The listing builds one solid part. Answer for the finished solid, in the listing's coordinates (mm). A direction names the side the tool comes from. Give positions to 0.01 mm unless a question says otherwise; leave off trailing zeros. Order: outer loops, then holes, each group sorted by start corner. A loop starts at its lowest first (then second) coordinate and runs counter-clockwise, first axis right, second up. Notation, with made-up numbers: (79.25, 16.25) - (130.25, 16.25) arc R29 ccw to (130.25, 46.25) - close; hole circle Ø7 at (13.25, 4). An arc over 180 degrees is marked (long way). Answer as a JSON object with one key per item and string values. Group by question number.
Q1. A cutting plane is placed at B-B, the plane y = 245.5. Give the vertices of the cut face in (x, z) (3 decimals), and give its area (3 significant figures).
Q2. Given pin 1 (6 mm diameter, centred on y = -110.93, z = 0, fed in from -X), flat-ended and moving along its own axis, determine where the tip first touches the part or whether it passes through.
Q3. For faces 1 (the face through (0, 5, 12.7)), 2 (the face through (22.225, 5, 0)), determine the directions among +Z, -Z, +X, -X, +Y, -Y from which every point of the face is accessible in a straight line to the end or side of a thin tool.
Q4. The mould has two halves that part along X. Classify faces 3 (the face through (0, -381, -10)), 4 (the face through (25.4, 5, 0)), 5 (the face through (-22.225, 5, 0)): released by +X, released by -X, zero draft, split by the parting line, or undercut.
Q5. A cutting plane is placed at A-A, the plane x = 1. Give the vertices of the cut face in (y, z) (3 decimals).
Q6. Consider line 1 (Y direction, x = -12.7, z = -10.75); line 2 (Z direction, x = 20, y = 268) (3 decimals); line 3 (X direction, y = 231.5, z = 1.5) (3 decimals). Determine where each line is inside the solid, lowest interval first.
from build123d import *

# Parameters (mm, degrees)
SKETCH1_W               = 50.8
SKETCH1_H               = 25.4
BOSS_EXTRUDE1_DEPTH     = 381
SHELL1_T                = -3.175
SKETCH4_R               = 2.38125
CUT_EXTRUDE1_DEPTH      = 385.581499815
CUT_EXTRUDE2_DEPTH      = 383.689587002
CUT_EXTRUDE2_DEPTH_BACK = 383.689587002
SKETCH5_R               = 2.38125


with BuildPart() as part:
    # Sketch1 → Boss-Extrude1 (new, symmetric)
    with BuildSketch(Plane(origin=(0, 0, 0), x_dir=(1, 0, 0), z_dir=(0, 1, 0))):
        Rectangle(SKETCH1_W, SKETCH1_H)
    extrude(amount=BOSS_EXTRUDE1_DEPTH, both=True)

    # Shell1
    shell1_openings = [part.faces().sort_by_distance(p)[0] for p in [
        (0, 381, 0),
        (0, -381, 0),
    ]]
    offset(amount=SHELL1_T, openings=shell1_openings, kind=Kind.INTERSECTION)

    # Sketch4 → Cut-Extrude1 (cut, through all)
    with BuildSketch(Plane(origin=(25.4, 0, 0), x_dir=(0, 0, -1), z_dir=(1, 0, 0))):
        with Locations((0, 110.9345)):
            Circle(SKETCH4_R)
        with Locations((0, 98.2345)):
            Circle(SKETCH4_R)
        with Locations((0, 85.5345)):
            Circle(SKETCH4_R)
        with Locations(Location((0, -85.5345, 0), (0, 0, 180))):
            Circle(SKETCH4_R)
        with Locations(Location((0, -98.2345, 0), (0, 0, 180))):
            Circle(SKETCH4_R)
        with Locations(Location((0, -110.9345, 0), (0, 0, 180))):
            Circle(SKETCH4_R)
        with Locations((0, -12.7)):
            Circle(SKETCH4_R)
        with Locations((0, -38.1)):
            Circle(SKETCH4_R)
        with Locations(Location((0, 38.1, 0), (0, 0, 180))):
            Circle(SKETCH4_R)
        with Locations(Location((0, 12.7, 0), (0, 0, 180))):
            Circle(SKETCH4_R)
    extrude(amount=-CUT_EXTRUDE1_DEPTH, mode=Mode.SUBTRACT)

    # Sketch5 → Cut-Extrude2 (cut, two sides: drawn at the far end of the back side and taken through both)
    with BuildSketch(Plane.XY.offset(12.7).offset(-CUT_EXTRUDE2_DEPTH_BACK)):
        with Locations((-12.7, 368.3)):
            Circle(SKETCH5_R)
        with Locations((12.7, 368.3)):
            Circle(SKETCH5_R)
        with Locations((12.7, 342.9)):
            Circle(SKETCH5_R)
        with Locations((-12.7, 342.9)):
            Circle(SKETCH5_R)
        with Locations((-12.7, -342.9)):
            Circle(SKETCH5_R)
        with Locations((12.7, -342.9)):
            Circle(SKETCH5_R)
        with Locations((12.7, -368.3)):
            Circle(SKETCH5_R)
        with Locations((-12.7, -368.3)):
            Circle(SKETCH5_R)
    extrude(amount=CUT_EXTRUDE2_DEPTH + CUT_EXTRUDE2_DEPTH_BACK, mode=Mode.SUBTRACT)


solid = part.part
Reply:
{
 "1": {"outline": "(-25.4, -12.7) - (25.4, -12.7) - (25.4, 12.7) - (-25.4, 12.7) - close; hole (-22.225, -9.525) - (22.225, -9.525) - (22.225, 9.525) - (-22.225, 9.525) - close", "area": "444 mm^2"},
 "2": {"pin 1": "stops at x = -25.4"},
 "3": {"face 1": "+Z, +X, -X, +Y, -Y", "face 2": "+Y, -Y"},
 "4": {"face 3": "zero draft", "face 4": "released by +X", "face 5": "undercut"},
 "5": {"outline": "(-381, -12.7) - (381, -12.7) - (381, -9.525) - (-381, -9.525) - close; (-381, 9.525) - (381, 9.525) - (381, 12.7) - (-381, 12.7) - close"},
 "6": {"line 1": "y = -381 to -370.68, -365.92 to -345.28, -340.52 to 340.52, 345.28 to 365.92, 370.68 to 381", "line 2": "z = -12.7 to -9.525, 9.525 to 12.7", "line 3": "x = -25.4 to -22.225, 22.225 to 25.4"}
}
